```python
from build123d import *

# Parameters (mm, degrees)
SKETCH1_W           = 50.8
SKETCH1_H           = 50.8
BOSS_EXTRUDE1_DEPTH = 6.35
SKETCH2_W           = 31.75
SKETCH2_H           = 31.75
BOSS_EXTRUDE2_DEPTH = 25.4
SKETCH3_W           = 50.8
SKETCH3_H           = 50.8
BOSS_EXTRUDE3_DEPTH = 6.35
SKETCH4_W           = 25.4
SKETCH4_H           = 25.4
CUT_EXTRUDE1_DEPTH  = 39.1
SKETCH5_R           = 2.38125
CUT_EXTRUDE2_DEPTH  = 39.1
CIRPATTERN1_COUNT   = 4
SCALE1_SCALE        = 1.02


with BuildPart() as part:
    # Sketch1 → Boss-Extrude1 (new body)
    with BuildSketch(Plane(origin=(0, 0, 0), x_dir=(1, 0, 0), z_dir=(0, 1, 0))):
        Rectangle(SKETCH1_W, SKETCH1_H)
    extrude(amount=BOSS_EXTRUDE1_DEPTH)

    # Sketch2 → Boss-Extrude2 (add)
    with BuildSketch(Plane(origin=(0, 6.35, 0), x_dir=(1, 0, 0), z_dir=(0, 1, 0))):
        Rectangle(SKETCH2_W, SKETCH2_H)
    extrude(amount=BOSS_EXTRUDE2_DEPTH)

    # Sketch3 → Boss-Extrude3 (add)
    with BuildSketch(Plane(origin=(0, 31.75, 0), x_dir=(1, 0, 0), z_dir=(0, 1, 0))):
        Rectangle(SKETCH3_W, SKETCH3_H)
    extrude(amount=BOSS_EXTRUDE3_DEPTH)

    # Sketch4 → Cut-Extrude1 (cut, through all)
    with BuildSketch(Plane(origin=(0, 38.1, 0), x_dir=(1, 0, 0), z_dir=(0, 1, 0))):
        Rectangle(SKETCH4_W, SKETCH4_H)
    extrude(amount=-CUT_EXTRUDE1_DEPTH, mode=Mode.SUBTRACT)

    # Sketch5 → Cut-Extrude2 (cut, through all)
    with BuildSketch(Plane(origin=(0, 38.1, 0), x_dir=(1, 0, 0), z_dir=(0, 1, 0))):
        with Locations((0, -20.6375)):
            Circle(SKETCH5_R)
    cut_extrude2 = extrude(amount=-CUT_EXTRUDE2_DEPTH, mode=Mode.SUBTRACT)

    # CirPattern1: Cut-Extrude2 ×4 about axis
    cirpattern1_axis = Axis((0, 0, 0), (0, 1, 0))
    for i in range(1, CIRPATTERN1_COUNT):
        add(cut_extrude2.rotate(cirpattern1_axis, i * 360 / CIRPATTERN1_COUNT), mode=Mode.SUBTRACT)


with BuildPart() as part_1:
    # Scale1: scaled about (0, 19.05, 0)
    add(part.part.scale(SCALE1_SCALE).moved(Location((0, -0.381, 0))))


solid = part_1.part
```
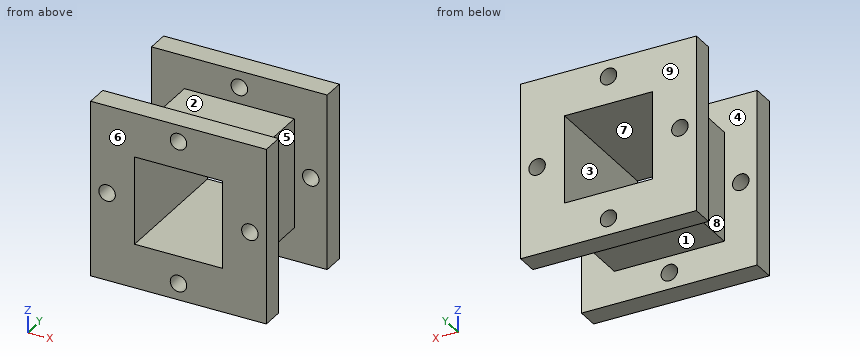
Input: part model. Units: mm. Frame: model coordinates. Face numbers are marked on the shaded views. A direction names the side the tool comes from. Coordinates: 2 decimals unless noted, no trailing zeros. Loops run counter-clockwise (first coordinate to the right, second up) from the corner with the lowest first, then second, coordinate; pieces in that order, holes last. Notation, with made-up numbers: M 70,-30.5 L 128,-30.5 A17 ccw 128,-10.5 Z; hole C -16.5,37 d3. An arc over 180 degrees is marked long. Answer in a Markdown table with one row per item.
1. First-contact query: pin 1 (5 mm diameter, centred on x = -12.5, y = 14.5, fed in from +Z); pin 2 (6 mm diameter, centred on y = 19, z = 2.5, fed in from -X); pin 3 (8 mm diameter, centred on x = -6.5, y = 20.5, fed in from -Z); pin 4 (3 mm diameter, centred on x = -21.05, z = 0, fed in from -Y). Flat tips, straight axial feed; report the tip coordinate or a pass-through.
Response:
| item | result |
|---|---|
| pin 1 | stops at z = 16.19 |
| pin 2 | stops at x = -16.19 |
| pin 3 | stops at z = -16.19 |
| pin 4 | passes through |
2. Section B-B, the plane z = -17. Output: boundary loops of the cut face in (x, y).
Response:
| item | result |
|---|---|
| outline | M -25.91,-0.38 L 25.91,-0.38 L 25.91,6.1 L -25.91,6.1 Z; M -25.91,32 L 25.91,32 L 25.91,38.48 L -25.91,38.48 Z |
3. Draft query along Y for the marked faces 6, 7, 8 and 9. Return one class per face: pulls with the +Y half, pulls with the -Y half, needs draft (parallel to the pull), parting line crosses it, or undercut.
Response:
| item | result |
|---|---|
| face 6 | pulls with the -Y half |
| face 7 | needs draft |
| face 8 | undercut |
| face 9 | pulls with the +Y half |
4. Section A-A, the plane x = -11. Output: boundary loops of the cut face in (y, z), then the cut area to 3 significant figures.
Response:
| item | result |
|---|---|
| outline | M -0.38,-25.91 L 6.1,-25.91 L 6.1,-16.19 L 32,-16.19 L 32,-25.91 L 38.48,-25.91 L 38.48,-12.95 L -0.38,-12.95 Z; M -0.38,12.95 L 38.48,12.95 L 38.48,25.91 L 32,25.91 L 32,16.19 L 6.1,16.19 L 6.1,25.91 L -0.38,25.91 Z |
| area | 503 mm2 |
5. Section D-D, the plane z = 0. Count the separate pieces of the cut face and the enclosed holes in it, then the cut area to 3 significant figures.
Response:
| item | result |
|---|---|
| separate pieces | 6 |
| enclosed holes | 0 |
| area | 378 mm2 |
6. Reachability of the marked faces 1, 2, 3, 4 and 5 from +Z, -Z, +X, -X, +Y, -Y: full face, straight path, thin tool, end or side. Return the list, or none.
Response:
| item | result |
|---|---|
| face 1 | -Z, +X, -X |
| face 2 | +Z, +X, -X |
| face 3 | +Y, -Y |
| face 4 | none |
| face 5 | +Z, -Z, +X |
7. Material intervals for line 1 (X direction, y = 33.5, z = 0); line 2 (X direction, y = 14, z = -10.5), sorted ascending.
Response:
| item | result |
|---|---|
| line 1 | x = -25.91 to -23.48, -18.62 to -12.95, 12.95 to 18.62, 23.48 to 25.91 |
| line 2 | x = -16.19 to -12.95, 12.95 to 16.19 |
8. Section C-C, the plane y = 22.5. Output: boundary loops of the cut face in (x, z), then the cut area to 3 significant figures.
Response:
| item | result |
|---|---|
| outline | M -16.19,-16.19 L 16.19,-16.19 L 16.19,16.19 L -16.19,16.19 Z; hole M -12.95,-12.95 L 12.95,-12.95 L 12.95,12.95 L -12.95,12.95 Z |
| area | 378 mm2 |
